```python
from build123d import *

# Parameters (mm, degrees)
RESSALTO_EXTRUS_O1_DEPTH                = 4
FURO_ROSCADO_DE_M21_D                   = 1.6
FURO_ROSCADO_PARA_CONDU_TE_DE_M4X0_71_D = 4.2


with BuildPart() as part:
    # Esboço1 → Ressalto-extrusão1 (new body)
    with BuildSketch(Plane.XY):
        with BuildLine():
            Line((-5.5, 0), (-5.5, -23))
            Line((-5.5, -23), (5.5, -23))
            Line((5.5, -23), (5.5, 0))
            ThreePointArc((5.5, 0), (0, 5.5), (-5.5, 0))
        make_face()
    extrude(amount=RESSALTO_EXTRUS_O1_DEPTH)

    # Furo roscado de M21 (through all)
    with Locations(Plane(origin=(-4, -20.5, 4), x_dir=(1, 0, 0), z_dir=(0, 0, 1))):
        with Locations((0, 0), (8, 0)):
            Hole(FURO_ROSCADO_DE_M21_D / 2)

    # Furo roscado para conduíte de M4x0.71 (through all)
    with Locations(Plane.XY.offset(4)):
        with Locations((0, 0)):
            Hole(FURO_ROSCADO_PARA_CONDU_TE_DE_M4X0_71_D / 2)


solid = part.part
```
Input: part model. Units: mm. Frame: model coordinates. Give positions to 0.01 mm unless a question says otherwise; leave off trailing zeros. Loops run counter-clockwise (first coordinate to the right, second up) from the corner with the lowest first, then second, coordinate; pieces in that order, holes last. Notation, with made-up numbers: M -10,3.5 L -1,3.5 A31 ccw -1,34.5 Z; hole C 70,29.25 d4. An arc over 180 degrees is marked long. Answer as CSV lines item,"result". Start each with the question number.
1. Section B-B on x = 0. Return loops of the section in (y, z).
2. Section C-C on z = 1. Return loops of the section in (x, y).
3. Section D-D on y = 1.5. Return loops of the section in (x, z).
4. Section A-A on y = -20.5. Return loops of the section in (x, z), plus the area to 3 significant figures.
5. Pull-direction query (Y, two-part tool) for faces 1 (the face through (-2.003, 0.631, 1.972)), 2 (the face through (0.1, 5.5, 2)), 3 (the face through (-5.5, -11, 2)); classes: released by +Y, released by -Y, zero draft, split by the parting line, or undercut.
6. Line query: L1, parallel to Y at x = 0, z = 2.1; L2, parallel to Y at x = -4, z = 2.2; L3, parallel to X at y = -1, z = 2.5. Output: solid intervals per line, ascending.
7. Pin query (flat end, axial travel): P1, Ø2.5, axis at x = 0, y = 0, coming from the +Z side. Return the tip coordinate at first contact, or that it passes through.
Computed values:
1,outline,"M -23,0 L -2.1,0 L -2.1,4 L -23,4 Z; M 2.1,0 L 5.5,0 L 5.5,4 L 2.1,4 Z"
2,outline,"M -5.5,-23 L 5.5,-23 L 5.5,0 A5.5 ccw -5.5,0 Z; hole C -4,-20.5 d1.6; hole C 0,0 d4.2; hole C 4,-20.5 d1.6"
3,outline,"M -5.29,0 L -1.47,0 L -1.47,4 L -5.29,4 Z; M 1.47,0 L 5.29,0 L 5.29,4 L 1.47,4 Z"
4,outline,"M -5.5,0 L -4.8,0 L -4.8,4 L -5.5,4 Z; M -3.2,0 L 3.2,0 L 3.2,4 L -3.2,4 Z; M 4.8,0 L 5.5,0 L 5.5,4 L 4.8,4 Z"
4,area,"31.2 mm²"
5,face 1,"undercut"
5,face 2,"released by +Y"
5,face 3,"zero draft"
6,L1,"y = -23 to -2.1, 2.1 to 5.5"
6,L2,"y = -23 to -21.3, -19.7 to 3.77"
6,L3,"x = -5.5 to -1.85, 1.85 to 5.5"
7,P1,"passes through"
